Geometry: see drawing. Coordinates: mm, zero at the bounding-box minimum. A direction names the side the tool comes from. Round coordinates to 2 decimals unless told otherwise and drop trailing zeros. Loops run counter-clockwise (first coordinate to the right, second up) from the corner with the lowest first, then second, coordinate; pieces in that order, holes last.
(1) Cut plane A-A, the plane x = 120. Output: boundary loops of the cut face in (y, z), and give its area (3 significant figures).
(2) Cut plane B-B, the plane z = 25. Output: boundary loops of the cut face in (x, y).
(3) Draft query along X for the marked faces 4, 5 and 6. Return one class per face: released by +X, released by -X, zero draft, split by the parting line, or undercut.
(4) Cut plane D-D, the plane x = 94. Output: boundary loops of the cut face in (y, z), and give its area (3 significant figures).
(5) First-contact query: pin 1 Ø1.5 at (x, z) = (41, 12) entering from -Y; pin 2 Ø1.5 at (x, z) = (18.5, 36.5) entering from +Y; pin 3 Ø18 at (x, y) = (120, 40) entering from -Z; pin 4 Ø8 at (x, z) = (118.5, 41) entering from +Y. Flat tips, straight axial feed; report the tip coordinate or a pass-through.
(6) Line query: line 1 (Y direction, x = 120, z = 38); line 2 (X direction, y = 39, z = 8); line 3 (Y direction, x = 20, z = 32). Output: solid intervals per line, ascending.
(7) Cut plane C-C, the plane x = 39. Output: boundary loops of the cut face in (y, z), and give its area (3 significant figures).
(8) Access query for the marked faces 1, 2 and 3. Directions: +Z, -Z, +X, -X, +Y, -Y. A direction counts if a zero-diameter tool reaches every point of the face in a straight line with its end or side. Return the directions, or none.
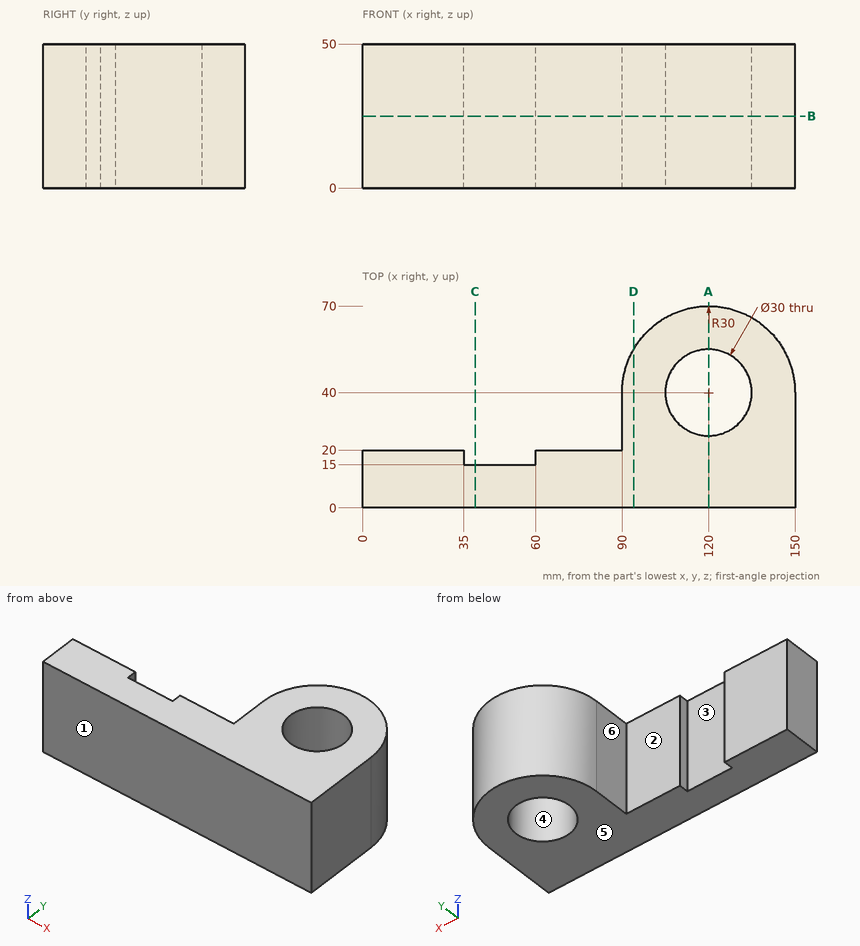
Reported:
1. outline: (0, 0) - (25, 0) - (25, 50) - (0, 50) - close; (55, 0) - (70, 0) - (70, 50) - (55, 50) - close
1. area: 2,000 mm2
2. outline: (0, 0) - (150, 0) - (150, 40) arc R30 ccw to (90, 40) - (90, 20) - (60, 20) - (60, 15) - (35, 15) - (35, 20) - (0, 20) - close; hole circle Ø30 at (120, 40)
3. face 4: undercut
3. face 5: zero draft
3. face 6: released by -X
4. outline: (0, 0) - (54.97, 0) - (54.97, 50) - (0, 50) - close
4. area: 2,750 mm2
5. pin 1: stops at y = 0
5. pin 2: stops at y = 20
5. pin 3: passes through
5. pin 4: stops at y = 70
6. line 1: y = 0 to 25, 55 to 70
6. line 2: x = 90 to 105.03, 134.97 to 150
6. line 3: y = 0 to 20
7. outline: (0, 0) - (15, 0) - (15, 50) - (0, 50) - close
7. area: 750 mm2
8. face 1: +Z, -Z, +X, -X, -Y
8. face 2: +Z, -Z, -X, +Y
8. face 3: +Z, -Z, +Y
